Source: CAD feature listing. Evaluate the final solid. Frame: model axes, mm. A direction names the side the tool comes from. Coordinates: 2 decimals unless noted, no trailing zeros. Order: outer loops, then holes, each group sorted by start corner. A loop starts at its lowest first (then second) coordinate and runs counter-clockwise, first axis right, second up. Notation, with made-up numbers: (-31, 21.5) - (-16, 21.5) arc R15 ccw to (-16, 33.5) - close; hole circle Ø4 at (72, 42.5). An arc over 180 degrees is marked (long way). One line per question, with ' | ' between items. Start each with the question number.
(1) Line query: line 1 along Y through (x, z) = (15, 0.8); line 2 along X through (y, z) = (30, 2.55); line 3 along X through (y, z) = (34.5, 3). Output: solid intervals per line, ascending.
(2) Section A-A (x = 111.5). Return the cut outline in (y, z).
(3) Contact query for flat-ended pins moving along their axis: P1, Ø6, axis at x = -1, y = -26.5, coming from the +Z side; P2, Ø3.5, axis at x = -15, y = -30, coming from the +Z side; P3, Ø2, axis at y = -5, z = 2, coming from the -X side; P4, Ø3, axis at x = 57, y = -22.5, coming from the -Z side. Output: stop coordinate, or through.
(4) Draft query along Y for faces 1 (the flat face through (-2, 40, 3)), 2 (the cylindrical face through (-148, -39, 3)), 3 (the cylindrical face through (149, 17, 3)). Return one class per face: +Y half, -Y half, draft (parallel to the pull), parting line (faces both ways), or undercut.
(5) Section C-C (x = -19.5). Return the cut outline in (y, z).
(6) Section B-B (z = 3). Count the separate pieces of the cut face and the enclosed holes in it, then the cut area to 3 significant figures.
(7) Access query for faces 4 (the flat face through (90, 0, 3)), 5 (the cylindrical face through (-92.85, -11.99, 2.96)), 6 (the flat face through (0, 30, 4)), 7 (the cylindrical face through (-149, 38, 3)). Directions: +Z, -Z, +X, -X, +Y, -Y. A direction counts if a zero-diameter tool reaches every point of the face in a straight line with its end or side. Return the directions, or none.
Autodesk Inventor part; units mm, degrees
ref_plane "YZ Plane" through (0, 0, 0) normal (1, 0, 0) x (0, 1, 0)
ref_plane "XZ Plane" through (0, 0, 0) normal (0, 1, 0) x (-1, 0, 0)
ref_plane "XY Plane" through (0, 0, 0) normal (0, 0, 1) x (1, 0, 0)
sketch "Esboço1" plane through (0, 0, 0) normal (0, 0, 1) x (1, 0, 0)
  line L0 (145, -40) -> (-145, -40)
  line L1 (-145, 40) -> (145, 40)
  line L2 (150, -40) -> (-150, 40) construction
  line L3 (-150, -40) -> (150, 40) construction
  line L4 (-145, -15) -> (-100, -15)
  line L5 (-90, -5) -> (-90, 5)
  line L6 (-100, 15) -> (-145, 15)
  line L7 (145, 15) -> (100, 15)
  line L8 (90, 5) -> (90, -5)
  line L9 (100, -15) -> (145, -15)
  line L10 (150, 35) -> (150, 20)
  line L11 (150, -20) -> (150, -35)
  line L12 (-150, -35) -> (-150, -20)
  line L13 (-150, 20) -> (-150, 35)
  arc A0 (100, 15) -> (90, 5) centre (100, 5) ccw
  arc A1 (90, -5) -> (100, -15) centre (100, -5) ccw
  arc A2 (-100, -15) -> (-90, -5) centre (-100, -5) ccw
  arc A3 (-90, 5) -> (-100, 15) centre (-100, 5) ccw
  arc A4 (150, 35) -> (145, 40) centre (145, 35) ccw
  arc A5 (145, 15) -> (150, 20) centre (145, 20) ccw
  arc A6 (150, -20) -> (145, -15) centre (145, -20) ccw
  arc A7 (145, -40) -> (150, -35) centre (145, -35) ccw
  arc A8 (-145, -15) -> (-150, -20) centre (-145, -20) ccw
  arc A9 (-150, -35) -> (-145, -40) centre (-145, -35) ccw
  arc A10 (-145, 40) -> (-150, 35) centre (-145, 35) ccw
  arc A11 (-150, 20) -> (-145, 15) centre (-145, 20) ccw
  point P0 (0, 0)
  point P1 (-150, -15)
  point P2 (-150, 15)
  point P3 (150, 15)
  dimension "d5" = 300
  dimension "d6" = 80
  dimension "d11" = 10
  dimension "d12" = 5
  dimension "d46" = 30
  dimension "d47" = 30
  dimension "d49" = 150
  dimension "d50" = 150
  dimension "d51" = 60
  dimension "d52" = 60
  dimension "d54" = 15
extrude "Extrusão1" add sketch "Esboço1" along normal blind 6
sketch "Esboço2" plane through (0, 0, 6) normal (0, 0, 1) x (1, 0, 0)
  line L0 (145, 40) -> (-145, 40)
  line L1 (25, -40) -> (-25, -40)
  line L2 (-25, 40) -> (25, 40)
  line L3 (25, -40) -> (-25, 40) construction
  line L4 (-25, -40) -> (25, 40) construction
  line L5 (-25, 20) -> (25, 20)
  line L6 (25, -20) -> (-25, -20)
  line L7 (-25, -40) -> (-25, -20)
  line L8 (-25, 20) -> (-25, 40)
  line L9 (25, 40) -> (25, 20)
  line L10 (25, -20) -> (25, -40)
  line L11 (-145, -40) -> (145, -40)
  point P0 (0, 0)
  dimension "d15" = 50
  dimension "d16" = 20
  dimension "d17" = 20
  dimension "d18" = 40
  dimension "d19" = 25
  dimension "d20" = 80
extrude "Extrusão2" cut sketch "Esboço2" against normal blind 2
sketch "Esboço3" plane through (0, 0, 4) normal (0, 0, 1) x (1, 0, 0)
  line L0 (25, 20) -> (-25, 20)
  line L1 (145, 40) -> (25, 40)
  line L2 (32.6697, 0) -> (-36.0886, 0) construction
  point P0 (0, 0)
  point P1 (15, 30)
  point P2 (-15, 30)
  point P3 (15, -30)
  point P4 (-15, -30)
  dimension "d23" = 10
  dimension "d24" = 20
  dimension "d25" = 15
  dimension "d26" = 30
  dimension "d27" = 10
hole "Furo1" at (15, 30, 4) at (-15, 30, 4) at (15, -30, 4) at (-15, -30, 4) direction (0, 0, -1) diameter 4 end through all
sketch "Esboço4" plane through (-145, 40, 0) normal (0, 1, 0) x (1, 0, 0)
  line L0 (290, -6) -> (170, -6)
  line L1 (290, 0) -> (0, 0)
  line L2 (295, 0) -> (295, -6)
  line L3 (145, -28.4495) -> (145, 21.5505) construction
  point P0 (145, 0)
  point P1 (275, -3)
  point P2 (145, 0)
  point P3 (15, -3)
  dimension "d35" = 3
  dimension "d36" = 6
  dimension "d37" = 20
  dimension "d38" = 50
hole "Furo2" at (130, 40, 3) at (-130, 40, 3) direction (0, -1, 0) diameter 4 end through all
equation "\"d47\" = d46"
equation "\"d52\" = d51"
equation "\"d18\" = -d17 + d20 - d16"
properties part number "Chassis" material "Plástico PC/ABS"
Response values:
1) line 1: y = -40 to -32, -28 to 28, 32 to 40 | line 2: x = -150 to -131.95, -128.05 to -17, -13 to 13, 17 to 128.05, 131.95 to 150 | line 3: x = -150 to -132, -128 to 128, 132 to 150
2) outline: (-40, 0) - (-15, 0) - (-15, 6) - (-40, 6) - close; (15, 0) - (40, 0) - (40, 6) - (15, 6) - close
3) P1: stops at z = 4 | P2: passes through | P3: stops at x = -90.05 | P4: stops at z = 0
4) face 1: +Y half | face 2: -Y half | face 3: undercut
5) outline: (-40, 0) - (40, 0) - (40, 4) - (20, 4) - (20, 6) - (-20, 6) - (-20, 4) - (-40, 4) - close
6) separate pieces: 5 | enclosed holes: 4 | area: 20,000 mm²
7) face 4: +Z, -Z, +X | face 5: +Z, -Z, -X | face 6: +Z, +Y | face 7: +Z, -Z, -X, +Y
